```python
from build123d import *

# Parameters (mm, degrees)
SKETCH2_W           = 148
SKETCH2_H           = 148
SKETCH2_R           = 3.5
SKETCH2_R_2         = 2.5
BOSS_EXTRUDE1_DEPTH = 3
FILLET1_R           = 40
CHAMFER1_SIZE       = 1.5
SKETCH3_W           = 25.243080612
SKETCH3_H           = 38.292469741
BOSS_EXTRUDE2_DEPTH = 3


with BuildPart() as part:
    # Sketch2 → Boss-Extrude1 (new body)
    with BuildSketch(Plane(origin=(0, 0, 0), x_dir=(1, 0, 0), z_dir=(0, 1, 0))):
        with Locations((50, -50)):
            Rectangle(SKETCH2_W, SKETCH2_H)
        with Locations(Location((0, 0, 0), (0, 0, 270))):
            Circle(SKETCH2_R, mode=Mode.SUBTRACT)
        with Locations(Location((0, -100, 0), (0, 0, 270))):
            Circle(SKETCH2_R, mode=Mode.SUBTRACT)
        with Locations(Location((100, 0, 0), (0, 0, 270))):
            Circle(SKETCH2_R, mode=Mode.SUBTRACT)
        with Locations(Location((100, -100, 0), (0, 0, 270))):
            Circle(SKETCH2_R, mode=Mode.SUBTRACT)
        with Locations(Location((50, -0.904618286, 0), (0, 0, 270))):
            Circle(SKETCH2_R_2, mode=Mode.SUBTRACT)
        with Locations(Location((50, -14.904618286, 0), (0, 0, 270))):
            Circle(SKETCH2_R_2, mode=Mode.SUBTRACT)
        with Locations(Location((50, -99.095381714, 0), (0, 0, 90))):
            Circle(SKETCH2_R_2, mode=Mode.SUBTRACT)
        with Locations(Location((50, -85.095381714, 0), (0, 0, 90))):
            Circle(SKETCH2_R_2, mode=Mode.SUBTRACT)
        with BuildLine():
            Line((-15.182460642, -21.358338014), (-15.182460642, -80.245012021))
            ThreePointArc((-15.182460642, -80.245012021), (-13.330510939, -83.016650619), (-10.061140298, -82.366332365))
            Line((-10.061140298, -82.366332365), (20.183871723, -52.121320344))
            ThreePointArc((20.183871723, -52.121320344), (21.062273515, -49.959169765), (20.125348516, -47.821728214))
            Line((20.125348516, -47.821728214), (-10.119663505, -19.180066228))
            ThreePointArc((-10.119663505, -19.180066228), (-13.368126824, -18.602581184), (-15.182460642, -21.358338014))
        make_face(mode=Mode.SUBTRACT)
        with BuildLine():
            Line((110.061140298, -82.366332365), (79.816128277, -52.121320344))
            ThreePointArc((79.816128277, -52.121320344), (78.937726485, -49.959169765), (79.874651484, -47.821728214))
            Line((79.874651484, -47.821728214), (110.119663505, -19.180066228))
            ThreePointArc((110.119663505, -19.180066228), (113.368126824, -18.602581184), (115.182460642, -21.358338014))
            Line((115.182460642, -21.358338014), (115.182460642, -80.245012021))
            ThreePointArc((115.182460642, -80.245012021), (113.330510939, -83.016650619), (110.061140298, -82.366332365))
        make_face(mode=Mode.SUBTRACT)
        with BuildLine():
            Line((5.995336985, -21.301386572), (15.004028172, -30.310077759))
            ThreePointArc((15.004028172, -30.310077759), (18.273398813, -30.960396013), (20.125348516, -28.188757415))
            Line((20.125348516, -28.188757415), (20.125348516, -10.171375041))
            ThreePointArc((20.125348516, -10.171375041), (18.273398813, -7.399736444), (15.004028172, -8.050054698))
            Line((15.004028172, -8.050054698), (5.995336985, -17.058745885))
            ThreePointArc((5.995336985, -17.058745885), (5.116657329, -19.180066228), (5.995336985, -21.301386572))
        make_face(mode=Mode.SUBTRACT)
        with BuildLine():
            Line((5.995336985, -78.698613428), (15.004028172, -69.689922241))
            ThreePointArc((15.004028172, -69.689922241), (18.273398813, -69.039603987), (20.125348516, -71.811242585))
            Line((20.125348516, -71.811242585), (20.125348516, -89.828624959))
            ThreePointArc((20.125348516, -89.828624959), (18.273398813, -92.600263556), (15.004028172, -91.949945302))
            Line((15.004028172, -91.949945302), (5.995336985, -82.941254115))
            ThreePointArc((5.995336985, -82.941254115), (5.116657329, -80.819933772), (5.995336985, -78.698613428))
        make_face(mode=Mode.SUBTRACT)
        with BuildLine():
            Line((79.874651484, -71.811242585), (79.874651484, -89.828624959))
            ThreePointArc((79.874651484, -89.828624959), (81.726601187, -92.600263556), (84.995971828, -91.949945302))
            Line((84.995971828, -91.949945302), (94.004663015, -82.941254115))
            ThreePointArc((94.004663015, -82.941254115), (94.883342671, -80.819933772), (94.004663015, -78.698613428))
            Line((94.004663015, -78.698613428), (84.995971828, -69.689922241))
            ThreePointArc((84.995971828, -69.689922241), (81.726601187, -69.039603987), (79.874651484, -71.811242585))
        make_face(mode=Mode.SUBTRACT)
        with BuildLine():
            Line((94.004663015, -21.301386572), (84.995971828, -30.310077759))
            ThreePointArc((84.995971828, -30.310077759), (81.726601187, -30.960396013), (79.874651484, -28.188757415))
            Line((79.874651484, -28.188757415), (79.874651484, -10.171375041))
            ThreePointArc((79.874651484, -10.171375041), (81.726601187, -7.399736444), (84.995971828, -8.050054698))
            Line((84.995971828, -8.050054698), (94.004663015, -17.058745885))
            ThreePointArc((94.004663015, -17.058745885), (94.883342671, -19.180066228), (94.004663015, -21.301386572))
        make_face(mode=Mode.SUBTRACT)
    extrude(amount=BOSS_EXTRUDE1_DEPTH)

    # Fillet1
    fillet1_edges = [part.edges().sort_by_distance(p)[0] for p in [
        (124, 1.5, 124),
        (-24, 1.5, 124),
        (-24, 1.5, -24),
        (124, 1.5, -24),
    ]]
    fillet(fillet1_edges, radius=FILLET1_R)

    # Chamfer1
    chamfer1_edges = [part.edges().sort_by_distance(p)[0] for p in [
        (50, 0, -1.595381714),
        (50, 0, 12.404618286),
        (50, 0, 101.595381714),
        (50, 0, 87.595381714),
    ]]
    chamfer(chamfer1_edges, length=CHAMFER1_SIZE)

    # Sketch3 → Boss-Extrude2 (add)
    with BuildSketch(Plane(origin=(0, 3, 0), x_dir=(1, 0, 0), z_dir=(0, 1, 0))):
        with Locations((50.641773236, -8.177777461)):
            Rectangle(SKETCH3_W, SKETCH3_H)
    extrude(amount=-BOSS_EXTRUDE2_DEPTH)


solid = part.part
```
Can you work these out from the model? Positions are in its coordinate system, mm. A direction names the side the tool comes from. Give positions to 0.01 mm unless a question says otherwise; leave off trailing zeros. Order: outer loops, then holes, each group sorted by start corner. A loop starts at its lowest first (then second) coordinate and runs counter-clockwise, first axis right, second up. Notation, with made-up numbers: (49.25, 86) - (64.25, 86) arc R20 cw to (64.25, 96) - close; hole circle Ø9 at (-37, 70.25). An arc over 180 degrees is marked (long way). Use a Markdown table: item, result. Add a question column.
Q1. If we section it at D-D on z = 0: Write out the boundary of the cut face in (x, y), plus the area to 3 significant figures.
Q2. If we section it at A-A on x = 50: Write out the boundary of the cut face in (y, z), plus the area to 4 significant figures.
Q3. On a 3-axis mill with a long thin cutter (end or side, diameter ignored), from which of +Z, -Z, +X, -X, +Y, -Y can I reach the whole of each face in a straight line? I mean faces 5 (the flat face through (89.563, 1.479, 25.743)), 6 (the cylindrical face through (111.972, 1.521, -12.594)). Say none if no direction works.
Q4. If we mould it in two halves opening along X, with no side actions, what happens to faces 1 (the cylindrical face through (111.972, 1.521, 112.594)), 2 (the cylindrical face through (-12.594, 1.521, 111.972)), 3 (the flat face through (4.85, 1.479, 67.456)), 4 (the cylindrical face through (-1.341, 1.479, 103.233))? For each: released by +X, released by -X, zero draft, split by the parting line, or undercut.
Q5. Please list where these lines run through material, in increasing order: line 1 along Z through (x, y) = (50, 2.2); line 2 along X through (y, z) = (0.3, 44); line 3 along X through (y, z) = (1.85, 17).
Q6. I'm going to push flat-ended pins straight in: pin 1 (6 mm diameter, centred on x = 17, z = 91.5, fed in from +Y); pin 2 (1.5 mm diameter, centred on y = 0.5, z = 88.5, fed in from -X); pin 3 (6.5 mm diameter, centred on x = 50, z = 85.1, fed in from -Y). Where does each tip first touch, or does it pass through?
Q7. If we section it at C-C on x = -13: Write out the boundary of the cut face in (y, z).
Q8. If we section it at B-B on z = 41: Write out the boundary of the cut face in (x, y).
Answers follow:
| question | item | result |
|---|---|---|
| 1 | outline | (-20.66, 0) - (-3.5, 0) - (-3.5, 3) - (-20.66, 3) - close; (3.5, 0) - (96.5, 0) - (96.5, 3) - (3.5, 3) - close; (103.5, 0) - (120.66, 0) - (120.66, 3) - (103.5, 3) - close |
| 1 | area | 382 mm^2 |
| 2 | outline | (0, -24) - (3, -24) - (3, 82.6) - (1.5, 82.6) - (0, 81.1) - close; (0, 89.1) - (1.5, 87.6) - (3, 87.6) - (3, 96.6) - (1.5, 96.6) - (0, 95.1) - close; (0, 103.1) - (1.5, 101.6) - (3, 101.6) - (3, 124) - (0, 124) - close |
| 2 | area | 409.5 mm^2 |
| 3 | face 5 | +Y, -Y |
| 3 | face 6 | -Z, +X, +Y, -Y |
| 4 | face 1 | released by +X |
| 4 | face 2 | released by -X |
| 4 | face 3 | undercut |
| 4 | face 4 | undercut |
| 5 | line 1 | z = -24 to 82.6, 87.6 to 96.6, 101.6 to 124 |
| 5 | line 2 | x = -24 to -15.18, 16.09 to 83.91, 115.18 to 124 |
| 5 | line 3 | x = -24 to 6.05, 20.13 to 79.87, 93.95 to 124 |
| 6 | pin 1 | stops at y = 3 |
| 6 | pin 2 | stops at x = -23.82 |
| 6 | pin 3 | stops at y = 0.75 |
| 7 | outline | (0, -11.55) - (3, -11.55) - (3, 18.47) - (0, 18.47) - close; (0, 83.13) - (3, 83.13) - (3, 111.55) - (0, 111.55) - close |
| 8 | outline | (-24, 0) - (-15.18, 0) - (-15.18, 3) - (-24, 3) - close; (12.92, 0) - (87.08, 0) - (87.08, 3) - (12.92, 3) - close; (115.18, 0) - (124, 0) - (124, 3) - (115.18, 3) - close |
